```python
from build123d import *

# Parameters (mm, degrees)
CYLINDER237_R               = 1.5
CYLINDER237_DEPTH           = 20
CYLINDER237_PLACEMENT_ANGLE = 67.5
CYLINDER244_R               = 1.5
CYLINDER244_DEPTH           = 20
CYLINDER244_PLACEMENT_ANGLE = 112.500001
CYLINDER239_R               = 1.5
CYLINDER239_DEPTH           = 20
CYLINDER239_PLACEMENT_ANGLE = 157.5
CYLINDER242_R               = 1.5
CYLINDER242_DEPTH           = 20
CYLINDER242_PLACEMENT_ANGLE = 202.5
CYLINDER240_R               = 1.5
CYLINDER240_DEPTH           = 20
CYLINDER240_PLACEMENT_ANGLE = 112.500005
CYLINDER243_R               = 1.5
CYLINDER243_DEPTH           = 20
CYLINDER243_PLACEMENT_ANGLE = 67.5
CYLINDER238_R               = 1.5
CYLINDER238_DEPTH           = 20
CYLINDER238_PLACEMENT_ANGLE = 22.5
CYLINDER241_R               = 1.5
CYLINDER241_DEPTH           = 20
CYLINDER241_PLACEMENT_ANGLE = 22.5
TUBE024_R                   = 46
TUBE024_R_2                 = 32
TUBE024_DEPTH               = 3


with BuildPart() as obj1:
    # Cylinder237 → Cylinder237 (new body)
    with BuildSketch(Plane.XY):
        Circle(CYLINDER237_R)
    extrude(amount=CYLINDER237_DEPTH)


with BuildPart() as obj1_1:
    # Cylinder237 placement: moved
    add(obj1.part.moved(Location((13.39392, 32.335784, -22))).rotate(Axis((13.39392, 32.335784, -22), (0, 0, 1)), CYLINDER237_PLACEMENT_ANGLE))


with BuildPart() as obj2:
    # Cylinder244 → Cylinder244 (new body)
    with BuildSketch(Plane.XY):
        Circle(CYLINDER244_R)
    extrude(amount=CYLINDER244_DEPTH)


with BuildPart() as obj2_1:
    # Cylinder244 placement: moved
    add(obj2.part.moved(Location((-13.39392, 32.335784, -22))).rotate(Axis((-13.39392, 32.335784, -22), (0, 0, 1)), CYLINDER244_PLACEMENT_ANGLE))


with BuildPart() as obj3:
    # Cylinder239 → Cylinder239 (new body)
    with BuildSketch(Plane.XY):
        Circle(CYLINDER239_R)
    extrude(amount=CYLINDER239_DEPTH)


with BuildPart() as obj3_1:
    # Cylinder239 placement: moved
    add(obj3.part.moved(Location((-32.335784, 13.39392, -22))).rotate(Axis((-32.335784, 13.39392, -22), (0, 0, 1)), CYLINDER239_PLACEMENT_ANGLE))


with BuildPart() as obj4:
    # Cylinder242 → Cylinder242 (new body)
    with BuildSketch(Plane.XY):
        Circle(CYLINDER242_R)
    extrude(amount=CYLINDER242_DEPTH)


with BuildPart() as obj4_1:
    # Cylinder242 placement: moved
    add(obj4.part.moved(Location((-32.335784, -13.39392, -22))).rotate(Axis((-32.335784, -13.39392, -22), (0, 0, 1)), CYLINDER242_PLACEMENT_ANGLE))


with BuildPart() as obj5:
    # Cylinder240 → Cylinder240 (new body)
    with BuildSketch(Plane.XY):
        Circle(CYLINDER240_R)
    extrude(amount=CYLINDER240_DEPTH)


with BuildPart() as obj5_1:
    # Cylinder240 placement: moved
    add(obj5.part.moved(Location((-13.39392, -32.335784, -22))).rotate(Axis((-13.39392, -32.335784, -22), (0, 0, -1)), CYLINDER240_PLACEMENT_ANGLE))


with BuildPart() as obj6:
    # Cylinder243 → Cylinder243 (new body)
    with BuildSketch(Plane.XY):
        Circle(CYLINDER243_R)
    extrude(amount=CYLINDER243_DEPTH)


with BuildPart() as obj6_1:
    # Cylinder243 placement: moved
    add(obj6.part.moved(Location((13.39392, -32.335784, -22))).rotate(Axis((13.39392, -32.335784, -22), (0, 0, -1)), CYLINDER243_PLACEMENT_ANGLE))


with BuildPart() as obj7:
    # Cylinder238 → Cylinder238 (new body)
    with BuildSketch(Plane.XY):
        Circle(CYLINDER238_R)
    extrude(amount=CYLINDER238_DEPTH)


with BuildPart() as obj7_1:
    # Cylinder238 placement: moved
    add(obj7.part.moved(Location((32.335784, -13.39392, -22))).rotate(Axis((32.335784, -13.39392, -22), (0, 0, -1)), CYLINDER238_PLACEMENT_ANGLE))


with BuildPart() as compound223:
    # Cylinder241 → Cylinder241 (new body)
    with BuildSketch(Plane.XY):
        Circle(CYLINDER241_R)
    extrude(amount=CYLINDER241_DEPTH)


with BuildPart() as compound223_1:
    # Cylinder241 placement: moved
    add(compound223.part.moved(Location((32.335784, 13.39392, -22))).rotate(Axis((32.335784, 13.39392, -22), (0, 0, 1)), CYLINDER241_PLACEMENT_ANGLE))

    # Compound223: union obj1, obj2, obj3, obj4, obj5, obj6, obj7
    add(obj1_1.part)
    add(obj2_1.part)
    add(obj3_1.part)
    add(obj4_1.part)
    add(obj5_1.part)
    add(obj6_1.part)
    add(obj7_1.part)


with BuildPart() as compound223_2:
    # Compound223 placement: moved
    add(compound223_1.part.moved(Location((0, 0, 2))))


with BuildPart() as obj8:
    # Tube024 → Tube024 (new body)
    with BuildSketch(Plane.XY.offset(-18)):
        Circle(TUBE024_R)
        Circle(TUBE024_R_2, mode=Mode.SUBTRACT)
    extrude(amount=TUBE024_DEPTH)

    # Cut117: cut Compound223
    add(compound223_2.part, mode=Mode.SUBTRACT)


solid = obj8.part
```
Verification items for the finished model (mm, model axes). Round coordinates to 2 decimals unless told otherwise and drop trailing zeros. Write each loop counter-clockwise with the first axis right and the second up, starting at its lowest first coordinate (ties: lowest second). Pieces come first, ordered by that corner, then holes. Notation, with made-up numbers: (-30.5, 25.25) -> (-15.5, 25.25) arc R11 ccw to (-15.5, 42.25) -> close; hole circle Ø6 at (32.5, 83). An arc over 180 degrees is marked (long way). Write each question's results on one line, items separated by ' | '.
Q1. Draft check along Y on faces 1 (the face through (30.977, -12.76, -16.521)), 2 (the face through (-31, -10, -15)), 3 (the face through (-5.99, 45.61, -16.52)). Enter one of: released by +Y, released by -Y, zero draft, split by the parting line, or undercut.
Derived:
face 1: undercut | face 2: zero draft | face 3: split by the parting line
Q2. Thickness scan on probe 1 along X at (y, z) = (0.5, -17.35); probe 2 along X at (y, z) = (-10.5, -16.05); probe 3 along Y at (x, z) = (-4, -17). Record the ranges inside material, lowest first.
Derived:
probe 1: x = -46 to -32, 32 to 46 | probe 2: x = -44.79 to -30.23, 30.23 to 44.79 | probe 3: y = -45.83 to -31.75, 31.75 to 45.83
Q3. Sectioned sample at A-A, the plane y = 0. Record the boundary of the cut face in (x, z), and give its area (3 significant figures).
Derived:
outline: (-46, -18) -> (-32, -18) -> (-32, -15) -> (-46, -15) -> close; (32, -18) -> (46, -18) -> (46, -15) -> (32, -15) -> close | area: 84.0 mm²
Q4. Sectioned sample at C-C, the plane z = -15.7. Give the number of separate pieces and of enclosed holes in the cut face, and give its area (3 significant figures).
Derived:
separate pieces: 1 | enclosed holes: 9 | area: 3,370 mm²
Q5. Sectioned sample at D-D, the plane y = -38.5. Record the boundary of the cut face in (x, z), and give its area (3 significant figures).
Derived:
outline: (-25.17, -18) -> (25.17, -18) -> (25.17, -15) -> (-25.17, -15) -> close | area: 151 mm²
Q6. Go/stop test with flat-tipped pins: pin 1 Ø1.8 at (x, y) = (32.34, 13.39) entering from +Z; pin 2 Ø1.5 at (x, z) = (-26.5, -16.5) entering from +Y. Record where each tip stops, or that it passes through.
Derived:
pin 1: passes through | pin 2: stops at y = 38.12
